Work out the finished part from the listing and answer in its coordinate system (mm). Give positions to 0.01 mm unless a question says otherwise; leave off trailing zeros. Loops run counter-clockwise (first coordinate to the right, second up) from the corner with the lowest first, then second, coordinate; pieces in that order, holes last. Notation, with made-up numbers: M -38,37.25 L 17,37.25 A25 cw 17,68.25 Z; hole C 83.5,41 d6. An arc over 180 degrees is marked long. Answer in a Markdown table with one row per item. Add a question column.
from build123d import *

# Parameters (mm, degrees)
BOSS_EXTRUDE1_DEPTH = 6
SKETCH2_R           = 1.5
CUT_EXTRUDE1_DEPTH  = 10
FILLET1_DEPTH       = 6


with BuildPart() as part:
    # Sketch1 → Boss-Extrude1 (new body)
    with BuildSketch(Plane.XY):
        with BuildLine():
            Line((-11.842719282, 4), (-20, 4))
            Line((-20, 4), (-20, -4))
            Line((-20, -4), (-11.842719282, -4))
            ThreePointArc((-11.842719282, -4), (-12.5, 0), (-11.842719282, 4))
        make_face()
    extrude(amount=BOSS_EXTRUDE1_DEPTH)

    # Sketch2 → Cut-Extrude1 (cut)
    with BuildSketch(Plane.ZY.offset(20)):
        with Locations((3, 0)):
            Circle(SKETCH2_R)
    extrude(amount=-CUT_EXTRUDE1_DEPTH, mode=Mode.SUBTRACT)

    # Fillet1: read off the stored shape, not the designer's step
    # Fillet1 outline → Fillet1 (cut)
    with BuildSketch(Plane.XY):
        with BuildLine():
            Line((-20, -4), (-16, -4))
            ThreePointArc((-16, -4), (-18.828427125, -2.828427125), (-20, 0))
            Line((-20, 0), (-20, -4))
        make_face()
        with BuildLine():
            Line((-20, 4), (-20, 0))
            ThreePointArc((-20, 0), (-18.828427125, 2.828427125), (-16, 4))
            Line((-16, 4), (-20, 4))
        make_face()
    extrude(amount=FILLET1_DEPTH, mode=Mode.SUBTRACT)


solid = part.part
(1) Section D-D, the plane z = 5.75 is taken. Determine the outline of the cut face in (x, y).
(2) Section A-A, the plane z = 4.25 is taken. Determine the outline of the cut face in (x, y).
(3) The mould has two halves that part along Z. Classify faces 1 (the face through (-16, 0, 6)), 2 (the face through (-16.258, -0.575, 4.386)), 3 (the face through (-14, -4, 3)): pulls with the +Z half, pulls with the -Z half, needs draft (parallel to the pull), parting line crosses it, or undercut.
(4) Section C-C, the plane x = -14.5 is taken. Determine the outline of the cut face in (y, z).
(5) Consider line 1 along Y through (x, z) = (-12.5, 3); line 2 along Z through (x, y) = (-17.5, 0); line 3 along Y through (x, z) = (-19, 2.5). Determine where each line is inside the solid, lowest interval first. Write a range as from..to.
(6) Section B-B, the plane y = 0.25 is taken. Determine the outline of the cut face in (x, z).
(7) Each of these flat-tipped pins is pushed along its axis until it touches: P1, Ø1, axis at y = 0.5, z = 1.5, coming from the +X side; P2, Ø2, axis at y = 1, z = 1.5, coming from the +X side; P3, Ø2.5, axis at y = 0, z = 3, coming from the -X side. Where does it stop, or does it pass through?
Numbers:
| question | item | result |
|---|---|---|
| 1 | outline | M -16,-4 L -11.84,-4 A12.5 cw -11.84,4 L -16,4 A4 ccw Z |
| 2 | outline | M -19.91,-0.83 A4 ccw -16,-4 L -11.84,-4 A12.5 cw -12.47,-0.83 Z; M -19.91,0.83 L -12.47,0.83 A12.5 cw -11.84,4 L -16,4 A4 ccw Z |
| 3 | face 1 | pulls with the +Z half |
| 3 | face 2 | undercut |
| 3 | face 3 | needs draft |
| 4 | outline | M -4,0 L 4,0 L 4,6 L -4,6 Z; hole C 0,3 d3 |
| 5 | line 1 | y = -4..-1.5, 1.5..4 |
| 5 | line 2 | z = 0..1.5, 4.5..6 |
| 5 | line 3 | y = -2.65..-1.41, 1.41..2.65 |
| 6 | outline | M -19.99,0 L -12.5,0 L -12.5,1.52 L -19.99,1.52 Z; M -19.99,4.48 L -12.5,4.48 L -12.5,6 L -19.99,6 Z |
| 7 | P1 | stops at x = -12.46 |
| 7 | P2 | stops at x = -12.34 |
| 7 | P3 | passes through |
